from build123d import *

# Parameters (mm, degrees)
F1_START = -3
F0_R     = 3.5
F1_DEPTH = 25
F0_R_2   = 11
F2_DEPTH = 28
F3_R     = 0.75
F4_DEPTH = 12.7
F5_SIZE  = 1


with BuildPart() as f1:
    # F0 (on Right) → F1 (new body)
    with BuildSketch(Plane.YZ.offset(F1_START)):
        Circle(F0_R)
    extrude(amount=-F1_DEPTH)

    # F0 (on Right) → F2 (join, symmetric)
    with BuildSketch(Plane.YZ):
        Circle(F0_R_2)
        Circle(F0_R, mode=Mode.SUBTRACT)
    extrude(amount=F2_DEPTH, both=True)

    # F3 (on Top) → F4 (cut)
    with BuildSketch(Plane.XY):
        Circle(F3_R)
    extrude(amount=F4_DEPTH, mode=Mode.SUBTRACT)

    # F5
    f5_edges = [f1.edges().sort_by_distance(p)[0] for p in [
        (28, -3.5, 0),
    ]]
    chamfer(f5_edges, length=F5_SIZE)


solid = f1.part
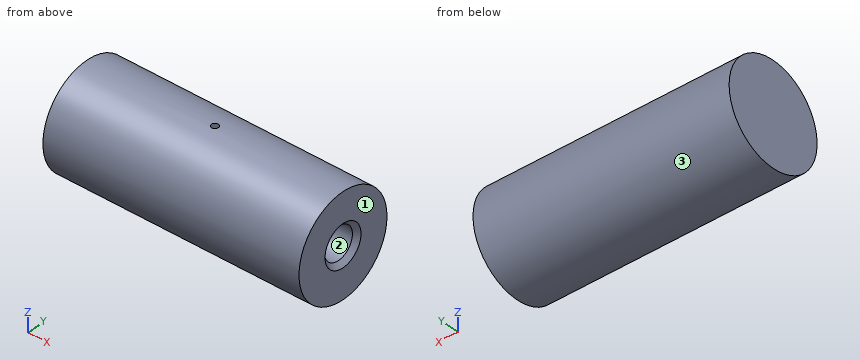
Build history of the part. All positions in model axes, mm. Face numbers are marked on the shaded views. Give positions to 0.01 mm unless a question says otherwise; leave off trailing zeros. Loops run counter-clockwise (first coordinate to the right, second up) from the corner with the lowest first, then second, coordinate; pieces in that order, holes last. Notation, with made-up numbers: (84, 14) - (99, 14) arc R20 ccw to (99, 48) - close; hole circle Ø7 at (-2, 38). An arc over 180 degrees is marked (long way). Write item = value, one per line. Start each with the question number.
1) Drop flat-ended pins along their axis: pin 1 Ø2 at (x, z) = (-5, 8) entering from -Y; pin 2 Ø2 at (x, y) = (-20.5, 7.5) entering from -Z; pin 3 Ø5.5 at (y, z) = (-1, 1) entering from +X. Give the stop position or say it passes through.
2) Band-saw the part on C-C on x = 18.5. Give the cut face in (y, z).
3) Pull direction Y, two halves, no side cores. Call the marked faces 1, 2 and 3: +Y half, -Y half, draft (parallel to the pull), parting line (faces both ways), or undercut.
4) Band-saw the part on B-B on z = 0. Give the cut face in (x, y).
5) Probe probe 1 along Z at (x, y) = (12, 0); probe 2 along Z at (x, y) = (-9.5, -0.5); probe 3 along Y at (x, z) = (0, 8.5). List the from-to ranges inside material, lowest first. Write a range as from..to.
6) Band-saw the part on A-A on y = 0. Give the cut face in (x, z).
7) Band-saw the part on D-D on z = 8. Give the cut face in (x, y), plus the area to 3 significant figures.
Final values:
q1.pin_1 = -8.49
q1.pin_2 = -8.87
q1.pin_3 = 27.66
q2.outline = circle Ø22 at (0, 0); hole circle Ø7 at (0, 0)
q3.face_1 = draft
q3.face_2 = undercut
q3.face_3 = parting line
q4.outline = (-28, -11) - (28, -11) - (28, -4.5) - (27, -3.5) - (-3, -3.5) - (-3, 3.5) - (27, 3.5) - (28, 4.5) - (28, 11) - (-28, 11) - close
q5.probe_1 = -11..-3.5, 3.5..11
q5.probe_2 = -10.99..10.99
q5.probe_3 = -6.98..-0.75, 0.75..6.98
q6.outline = (-28, -11) - (28, -11) - (28, -4.5) - (27, -3.5) - (-3, -3.5) - (-3, 3.5) - (-0.75, 3.5) - (-0.75, 11) - (-28, 11) - close; (0.75, 3.5) - (27, 3.5) - (28, 4.5) - (28, 11) - (0.75, 11) - close
q7.outline = (-28, -7.55) - (28, -7.55) - (28, 7.55) - (-28, 7.55) - close; hole circle Ø1.5 at (0, 0)
q7.area = 844 mm²
